from build123d import *

# Parameters (mm, degrees)
CROQUIS1_R              = 1.5
SALIENTE_EXTRUIR2_DEPTH = 2


with BuildPart() as part:
    # Croquis1 → Saliente-Extruir2 (new body)
    with BuildSketch(Plane(origin=(0, 0, 0), x_dir=(1, 0, 0), z_dir=(0, 1, 0))):
        with BuildLine():
            Line((10.296518832, -10.234095306), (10.296518832, -30.447615579))
            ThreePointArc((10.296518832, -30.447615579), (-0.203481168, 31.780682421), (-10.703481168, -30.447615579))
            Line((-10.703481168, -30.447615579), (-10.703481168, -10.234095306))
            Line((-10.703481168, -10.234095306), (10.296518832, -10.234095306))
        make_face()
        with Locations((-20.524295325, 20.101496578)):
            Circle(CROQUIS1_R, mode=Mode.SUBTRACT)
        with Locations((20.117332989, 20.101496578)):
            Circle(CROQUIS1_R, mode=Mode.SUBTRACT)
        with Locations((20.117332989, -20.540131736)):
            Circle(CROQUIS1_R, mode=Mode.SUBTRACT)
        with Locations((-20.524295325, -20.540131736)):
            Circle(CROQUIS1_R, mode=Mode.SUBTRACT)
    extrude(amount=SALIENTE_EXTRUIR2_DEPTH)


solid = part.part
Model file for the job. Use its own axes, mm. A direction names the side the tool comes from. Give positions to 0.01 mm unless a question says otherwise; leave off trailing zeros. Write each loop counter-clockwise with the first axis right and the second up, starting at its lowest first coordinate (ties: lowest second). Pieces come first, ordered by that corner, then holes. Notation, with made-up numbers: (-16, 3.25) -> (-8, 3.25) arc R15 ccw to (-8, 14.25) -> close; hole circle Ø10 at (-27.5, 23.25). An arc over 180 degrees is marked (long way). Write item = value, one per line.
(1) Slice it at A-A, the plane z = 14. Give the cut face in (x, y), then the cut area to 3 significant figures.
Determined:
outline = (-29.08, 0) -> (-10.7, 0) -> (-10.7, 2) -> (-29.08, 2) -> close; (10.3, 0) -> (28.68, 0) -> (28.68, 2) -> (10.3, 2) -> close
area = 73.5 mm2
(2) Mould opens along Z. For faces 3 (the face through (1.054, 0.986, -31.756)), 4 (the face through (18.62, 0.99, 20.47)), 5 (the face through (-1, 0, -1)), 6 (the face through (-19.094, 0.986, -20.552)) say: released by +Z, released by -Z, zero draft, split by the parting line, or undercut.
Determined:
face_3 = split by the parting line
face_4 = undercut
face_5 = zero draft
face_6 = undercut
(3) Slice it at B-B, the plane y = 1.1. Give the cut face in (x, z), then the cut area to 3 significant figures.
Determined:
outline = (-10.7, 10.23) -> (-10.7, 30.45) arc R32 ccw (long way) to (10.3, 30.45) -> (10.3, 10.23) -> close; hole circle Ø3 at (-20.52, -20.1); hole circle Ø3 at (-20.52, 20.54); hole circle Ø3 at (20.12, -20.1); hole circle Ø3 at (20.12, 20.54)
area = 2,740 mm2
(4) Probe line 1 along Z through (x, y) = (19, 1.25); line 2 along Z through (x, y) = (-21, 1.15); line 3 along X through (y, z) = (1.4, 28). List the from-to ranges inside material, lowest first.
Determined:
line_1 = -25.38 to -21.1, -19.1 to 19.54, 21.54 to 25.82
line_2 = -24.1 to -21.52, -18.68 to 19.12, 21.96 to 24.54
line_3 = -16.09 to -10.7, 10.3 to 15.68
(5) Tool access for faces 1 (the face through (0, 1, 10.234)), 2 (the face through (18.62, 0.99, -20.17)): list every direction of +Z, -Z, +X, -X, +Y, -Y with a clear straight run to the whole face (end or side of a thin tool).
Determined:
face_1 = +Z, +Y, -Y
face_2 = +Y, -Y
(6) Slice it at C-C, the plane x = -9.5. Give the cut face in (y, z), then the cut area to 3 significant figures.
Determined:
outline = (0, -30.4) -> (2, -30.4) -> (2, 10.23) -> (0, 10.23) -> close
area = 81.3 mm2
(7) Flat gauge pins, fed straight in: P1, Ø0.6, axis at x = 0, y = 1.5, coming from the +Z side; P2, Ø1, axis at y = 1, z = 16, coming from the -X side. Where does each tip first touch, or does it go through?
Determined:
P1 = 10.23
P2 = -28.32
(8) Slice it at D-D, the plane z = -6.5. Give the cut face in (x, y).
Determined:
outline = (-31.49, 0) -> (31.08, 0) -> (31.08, 2) -> (-31.49, 2) -> close
